Geometry check sheet. Reference: the model listing, model coordinates, mm. Give positions to 0.01 mm unless a question says otherwise; leave off trailing zeros. Put each result on its own line as item: value. Start each with the question number.
Q1. Section check A-A on z = 172.5. State how many separate pieces and enclosed holes the cut face has, then the cut area to 3 significant figures.
Q2. Go/stop test with flat-tipped pins: pin 1 (1.8 mm diameter, centred on y = 4.5, z = 348.5, fed in from +X); pin 2 (1.6 mm diameter, centred on x = 1.5, z = 355.5, fed in from -Y); pin 3 (1.3 mm diameter, centred on y = -4, z = 293.5, fed in from +X); pin 4 (5 mm diameter, centred on y = -1, z = 437, fed in from -X). Record where each tip stops, or that it passes through.
Q3. Material ranges on L1, parallel to Y at x = -7.25, z = 259; L2, parallel to Y at x = 8.25, z = 143.5; L3, parallel to Y at x = 0, z = 259, recorded low to high.
Autodesk Inventor part; units mm, degrees
ref_plane "Начальная плоскость" through (0, 0, 10) normal (0, 0, 1) x (1, 0, 0)
ref_plane "Конечная плоскость" through (0, 0, 500) normal (0, 0, 1) x (1, 0, 0)
ref_plane "РабПлоскость4" through (330, 0, 500) normal (0, 0, 1) x (1, 0, 0)
ref_plane "Начальная плоскость" through (0, 0, 10) normal (0, 0, 1) x (1, 0, 0)
ref_plane "Конечная плоскость" through (0, 0, 500) normal (0, 0, 1) x (1, 0, 0)
sketch "Эскиз" plane through (0, 0, 0) normal (0, 0, 1) x (1, 0, 0)
  line L0 (-14.4349, 0) -> (14.4349, 0)
  line L1 (0, -14) -> (0, 14)
  line L2 (0, 0) -> (7.5, 7.5) construction
  circle A0 centre (7.5, 7.5) radius 1.65 construction
  line L3 (5.85, 9.15) -> (9.15, 9.15)
  line L4 (9.15, 9.15) -> (9.15, 5.85)
  line L5 (9.15, 5.85) -> (5.85, 5.85)
  line L6 (5.85, 5.85) -> (5.85, 9.15)
  line L7 (3.235, 8.1636) -> (4.72, 9.9636)
  line L8 (4.7971, 10) -> (8.5, 10)
  line L9 (3.3121, 8) -> (4.95, 8)
  line L10 (4.95, 8) -> (4.95, 5.7985)
  line L11 (4.95, 5.7985) -> (2.6515, 3.5)
  line L12 (0, 3.5) -> (2.6515, 3.5)
  circle A1 centre (0, 0) radius 2.5
  line L13 (8.1636, 3.235) -> (9.9636, 4.72)
  line L14 (10, 4.7971) -> (10, 8.5)
  line L15 (8, 3.3121) -> (8, 4.95)
  line L16 (8, 4.95) -> (5.7985, 4.95)
  line L17 (5.7985, 4.95) -> (3.5, 2.6515)
  line L18 (3.5, 0) -> (3.5, 2.6515)
  arc A2 (10, 8.5) -> (8.5, 10) centre (8.5, 8.5) ccw
  line L19 (0, 0) -> (-7.5, 7.5) construction
  circle A3 centre (-7.5, 7.5) radius 1.65 construction
  line L20 (-5.85, 9.15) -> (-9.15, 9.15)
  line L21 (-9.15, 9.15) -> (-9.15, 5.85)
  line L22 (-9.15, 5.85) -> (-5.85, 5.85)
  line L23 (-5.85, 5.85) -> (-5.85, 9.15)
  line L24 (-3.235, 8.1636) -> (-4.72, 9.9636)
  line L25 (-4.7971, 10) -> (-8.5, 10)
  line L26 (-3.3121, 8) -> (-4.95, 8)
  line L27 (-4.95, 8) -> (-4.95, 5.7985)
  line L28 (-4.95, 5.7985) -> (-2.6515, 3.5)
  line L29 (0, 3.5) -> (-2.6515, 3.5)
  line L30 (-3.5, 0) -> (-3.5, 2.6515)
  line L31 (-5.7985, 4.95) -> (-3.5, 2.6515)
  line L32 (-8, 4.95) -> (-5.7985, 4.95)
  line L33 (-8, 3.3121) -> (-8, 4.95)
  line L34 (-8.1636, 3.235) -> (-9.9636, 4.72)
  line L35 (-10, 4.7971) -> (-10, 8.5)
  arc A4 (-8.5, 10) -> (-10, 8.5) centre (-8.5, 8.5) ccw
  line L36 (0, 14) -> (0, -14)
  line L37 (0, 0) -> (7.5, -7.5) construction
  circle A5 centre (7.5, -7.5) radius 1.65 construction
  line L38 (5.85, -9.15) -> (9.15, -9.15)
  line L39 (9.15, -9.15) -> (9.15, -5.85)
  line L40 (9.15, -5.85) -> (5.85, -5.85)
  line L41 (5.85, -5.85) -> (5.85, -9.15)
  line L42 (3.235, -8.1636) -> (4.72, -9.9636)
  line L43 (4.7971, -10) -> (8.5, -10)
  line L44 (3.3121, -8) -> (4.95, -8)
  line L45 (4.95, -8) -> (4.95, -5.7985)
  line L46 (4.95, -5.7985) -> (2.6515, -3.5)
  line L47 (0, -3.5) -> (2.6515, -3.5)
  line L48 (3.5, 0) -> (3.5, -2.6515)
  line L49 (5.7985, -4.95) -> (3.5, -2.6515)
  line L50 (8, -4.95) -> (5.7985, -4.95)
  line L51 (8, -3.3121) -> (8, -4.95)
  line L52 (8.1636, -3.235) -> (9.9636, -4.72)
  line L53 (10, -4.7971) -> (10, -8.5)
  arc A6 (8.5, -10) -> (10, -8.5) centre (8.5, -8.5) ccw
  line L54 (0, 0) -> (-7.5, -7.5) construction
  line L55 (-4.95, -8) -> (-4.95, -5.7985)
  line L56 (-3.3121, -8) -> (-4.95, -8)
  line L57 (-5.7985, -4.95) -> (-3.5, -2.6515)
  line L58 (-4.95, -5.7985) -> (-2.6515, -3.5)
  line L59 (-3.5, 0) -> (-3.5, -2.6515)
  line L60 (0, -3.5) -> (-2.6515, -3.5)
  circle A7 centre (-7.5, -7.5) radius 1.65 construction
  line L61 (-5.85, -5.85) -> (-5.85, -9.15)
  line L62 (-5.85, -9.15) -> (-9.15, -9.15)
  line L63 (-9.15, -9.15) -> (-9.15, -5.85)
  line L64 (-9.15, -5.85) -> (-5.85, -5.85)
  line L65 (-3.235, -8.1636) -> (-4.72, -9.9636)
  line L66 (-8, -4.95) -> (-5.7985, -4.95)
  line L67 (-8, -3.3121) -> (-8, -4.95)
  line L68 (-8.1636, -3.235) -> (-9.9636, -4.72)
  line L69 (-4.7971, -10) -> (-8.5, -10)
  line L70 (-10, -4.7971) -> (-10, -8.5)
  arc A8 (-10, -8.5) -> (-8.5, -10) centre (-8.5, -8.5) ccw
  arc A9 (3.235, 8.1636) -> (3.3121, 8) centre (3.3121, 8.1) ccw
  arc A10 (4.7971, 10) -> (4.72, 9.9636) centre (4.7971, 9.9) ccw
  arc A11 (8, 3.3121) -> (8.1636, 3.235) centre (8.1, 3.3121) ccw
  arc A12 (9.9636, 4.72) -> (10, 4.7971) centre (9.9, 4.7971) ccw
  arc A13 (-3.3121, 8) -> (-3.235, 8.1636) centre (-3.3121, 8.1) ccw
  arc A14 (-4.72, 9.9636) -> (-4.7971, 10) centre (-4.7971, 9.9) ccw
  arc A15 (-8.1636, 3.235) -> (-8, 3.3121) centre (-8.1, 3.3121) ccw
  arc A16 (-10, 4.7971) -> (-9.9636, 4.72) centre (-9.9, 4.7971) ccw
  arc A17 (-8, -3.3121) -> (-8.1636, -3.235) centre (-8.1, -3.3121) ccw
  arc A18 (-9.9636, -4.72) -> (-10, -4.7971) centre (-9.9, -4.7971) ccw
  arc A19 (-3.235, -8.1636) -> (-3.3121, -8) centre (-3.3121, -8.1) ccw
  arc A20 (-4.7971, -10) -> (-4.72, -9.9636) centre (-4.7971, -9.9) ccw
  arc A21 (4.72, -9.9636) -> (4.7971, -10) centre (4.7971, -9.9) ccw
  arc A22 (3.3121, -8) -> (3.235, -8.1636) centre (3.3121, -8.1) ccw
  arc A23 (8.1636, -3.235) -> (8, -3.3121) centre (8.1, -3.3121) ccw
  arc A24 (10, -4.7971) -> (9.9636, -4.72) centre (9.9, -4.7971) ccw
  point P0 (3.1, 8)
  point P1 (4.75, 10)
  point P2 (7.5, 9.15)
  point P3 (8, 3.1)
  point P4 (10, 4.75)
  point P5 (7.5, 5.85)
  point P6 (9.15, 7.5)
  point P7 (-3.1, 8)
  point P8 (-4.75, 10)
  point P9 (-7.5, 9.15)
  point P10 (-8, 3.1)
  point P11 (-10, 4.75)
  point P12 (-7.5, 5.85)
  point P13 (-9.15, 7.5)
  point P14 (3.1, -8)
  point P15 (4.75, -10)
  point P16 (7.5, -9.15)
  point P17 (8, -3.1)
  point P18 (10, -4.75)
  point P19 (7.5, -5.85)
  point P20 (9.15, -7.5)
  point P21 (-3.1, -8)
  point P22 (-7.5, -5.85)
  point P23 (-7.5, -9.15)
  point P24 (-9.15, -7.5)
  point P25 (-4.75, -10)
  point P26 (-8, -3.1)
  point P27 (-10, -4.75)
  dimension "d0" = 45
  dimension "d1" = 3.3
  dimension "d2" = 1.5
  dimension "d3" = 1.2
  dimension "d4" = 5
  dimension "d5" = 6.5
  dimension "d6" = 15
  dimension "d7" = 20
  dimension "d8" = 9.9
  dimension "d9" = 9.5
  dimension "d10" = 6.2
  dimension "d11" = 2
  dimension "d18" = 0.1
  dimension "d19" = 0.1
extrude "Тело" add sketch "Эскиз" along normal up to surface (490 mm away) from surface at 10 contours A1 L1 L12 L11 L10 L9 A9 L7 A10 L8 A2 L14 A12 L13 A11 L15 L16 L17 L18 L0 | L0 L48 L49 L50 L51 A23 L52 A24 L53 A6 L43 A21 L42 A22 L44 L45 L46 L47 L1 A1 | A1 L0 L30 L31 L32 L33 A15 L34 A16 L35 A4 L25 A14 L24 A13 L26 L27 L28 L29 L1 | L1 L60 L58 L55 L56 A19 L65 A20 L69 A8 L70 A18 L68 A17 L67 L66 L57 L59 L0 A1
sketch "Эскиз2" plane through (0, 0, 0) normal (0, 0, 1) x (1, 0, 0)
  line L0 (0, 0) -> (10, 0)
ref_plane "РабПлоскость3" through (0, 0, 0) normal (0, -1, 0) x (1, 0, 0)
sketch "Эскиз3" plane through (0, 0, 0) normal (0, -1, 0) x (1, 0, 0)
  line L0 (-2, 10) -> (12, 10)
  line L1 (-2, 500) -> (12, 500)
  dimension "d25" = 490
ref_plane "РабПлоскость4" through (330, 0, 500) normal (0, 0, 1) x (1, 0, 0)
split "Разделение1" plane through (330, 0, 500) removes the side toward (0, 0, 1)
ref_plane "РабПлоскость5" through (300, 0, 10) normal (0, 0, -1) x (-1, 0, 0)
split "Разделение2" plane through (300, 0, 10) removes the side toward (0, 0, -1)
ref_plane "РабПлоскость6" through (0, 40, -10) normal (0, 0, -1) x (-1, 0, 0)
split "Разделение3" plane through (0, 40, -10) removes the side toward (0, 0, -1)
properties part number "короткая палка" material "Алюминий 6061"
Results found:
1. separate pieces: 1
1. enclosed holes: 5
1. area: 115 mm^2
2. pin 1: stops at x = 10
2. pin 2: stops at y = -3.5
2. pin 3: stops at x = 9.88
2. pin 4: stops at x = -8.48
3. L1: y = -10 to -9.15, -5.85 to -4.95, 4.95 to 5.85, 9.15 to 10
3. L2: y = -10 to -9.15, -5.85 to -3.31, 3.31 to 5.85, 9.15 to 10
3. L3: y = -3.5 to -2.5, 2.5 to 3.5
